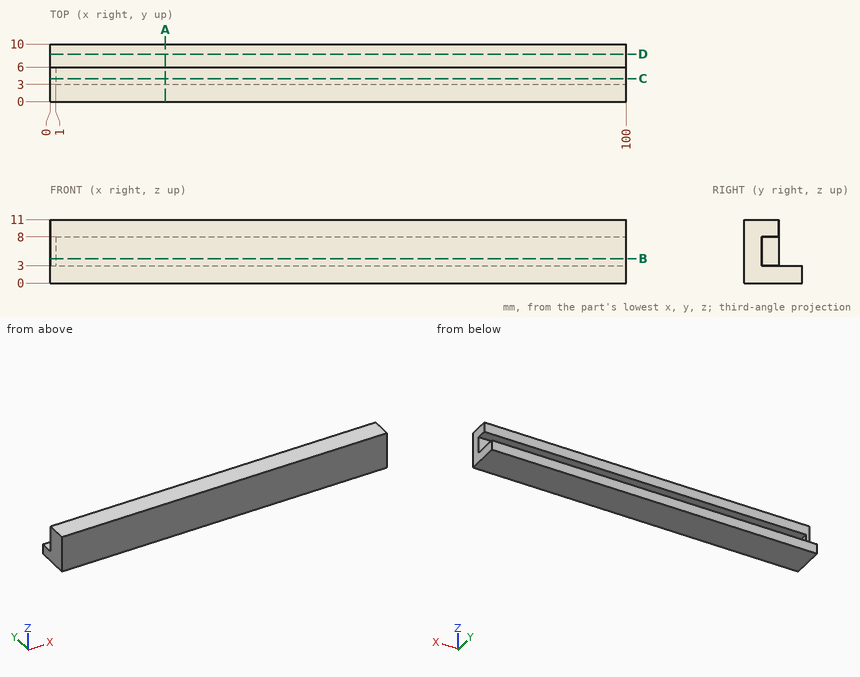
The drawing under review shows one solid part. Ordinate dimensions are in mm from its lowest x, y, z. Round coordinates to 2 decimals unless told otherwise and drop trailing zeros. Order: outer loops, then holes, each group sorted by start corner. A loop starts at its lowest first (then second) coordinate and runs counter-clockwise, first axis right, second up. Notation, with made-up numbers: (-9.5, 57) -> (10.5, 57) arc R15 ccw to (10.5, 79) -> close; hole circle Ø4 at (76, 33). An arc over 180 degrees is marked (long way). Use a Markdown table: item, result.
Q1. Clearance check with flat-ended pins moving along their axes: P1, Ø2.5, axis at x = 62, z = 4.5, coming from the +Y side; P2, Ø1.5, axis at y = 5, z = 5.5, coming from the +X side. State where each tip first meets the part, or that it passes through.
Values:
| item | result |
|---|---|
| P1 | stops at y = 3 |
| P2 | stops at x = 1 |
Q2. We need section D-D on y = 8.25. Write out the cut boundary in (x, z).
Values:
| item | result |
|---|---|
| outline | (0, 0) -> (100, 0) -> (100, 3) -> (0, 3) -> close |
Q3. We need section A-A on x = 20. Write out the cut boundary in (y, z), then the cut area to 3 significant figures.
Values:
| item | result |
|---|---|
| outline | (0, 0) -> (10, 0) -> (10, 3) -> (3, 3) -> (3, 8) -> (6, 8) -> (6, 11) -> (0, 11) -> close |
| area | 63.0 mm^2 |
Q4. For line 1 (Z direction, x = 55, y = 4); line 2 (X direction, y = 4.25, z = 7.75); line 3 (Z direction, x = 6.5, y = 9), list the stretches that pass through material, from the lowest coordinate up.
Values:
| item | result |
|---|---|
| line 1 | z = 0 to 3, 8 to 11 |
| line 2 | x = 0 to 1 |
| line 3 | z = 0 to 3 |
Q5. We need section B-B on z = 4.25. Write out the cut boundary in (x, y).
Values:
| item | result |
|---|---|
| outline | (0, 0) -> (100, 0) -> (100, 3) -> (1, 3) -> (1, 6) -> (0, 6) -> close |
Q6. We need section C-C on y = 4. Write out the cut boundary in (x, z), then the cut area to 3 significant figures.
Values:
| item | result |
|---|---|
| outline | (0, 0) -> (100, 0) -> (100, 3) -> (1, 3) -> (1, 8) -> (100, 8) -> (100, 11) -> (0, 11) -> close |
| area | 605 mm^2 |
